Build history of the part. All positions in model axes, mm. Face numbers are marked on the shaded views. A direction names the side the tool comes from. Round coordinates to 2 decimals unless told otherwise and drop trailing zeros. Loops run counter-clockwise (first coordinate to the right, second up) from the corner with the lowest first, then second, coordinate; pieces in that order, holes last. Notation, with made-up numbers: (79, -30) - (102, -30) arc R32 ccw to (102, -3) - close; hole circle Ø8 at (57.25, -31). An arc over 180 degrees is marked (long way). Use one line per item in the form item = value. Start each with the question number.
Q1. Saw through at A-A (x = 0). Give the cut face in (y, z).
Q2. Saw through at D-D (x = 12). Give the cut face in (y, z), then the cut area to 3 significant figures.
Q3. Mould opens along X. For the marked faces 1, 2 and 3 say: released by +X, released by -X, zero draft, split by the parting line, or undercut.
Q4. Saw through at B-B (z = 4). Give the cut face in (x, y).
Q5. Saw through at C-C (y = -9). Give the cut face in (x, z).
Q6. Pin check, flat tips, straight feed: pin 1 (6 mm diameter, centred on x = 32, y = 4.5, fed in from +Z); pin 2 (1 mm diameter, centred on y = -10.5, z = 8.5, fed in from -X); pin 3 (1.5 mm diameter, centred on x = 18, z = 13, fed in from -Y). Stop position of each tip, or through.
Q7. Drill centre lines: line 1 (Z direction, x = -38.5, y = 21.5); line 2 (X direction, y = 3, z = 10.75); line 3 (X direction, y = 16.5, z = 18.5). Where is each one in solid material? Low to high.
Q8. 3-axis set-ups, long thin cutter, end or side, ignore diameter. For the marked faces 4, 5 and 6: which of +Z, -Z, +X, -X, +Y, -Y reach the whole face in a straight line?
```python
from build123d import *

# Parameters (mm, degrees)
SKETCH1_R           = 50.8
BOSS_EXTRUDE1_DEPTH = 6.35
SKETCH2_R           = 19.05
BOSS_EXTRUDE2_DEPTH = 19.05
CUT_EXTRUDE1_DEPTH  = 25.4
SKETCH4_R           = 3.81


with BuildPart() as part:
    # Sketch1 → Boss-Extrude1 (new body)
    with BuildSketch(Plane.XY):
        Circle(SKETCH1_R)
    extrude(amount=BOSS_EXTRUDE1_DEPTH)

    # Sketch2 → Boss-Extrude2 (add)
    with BuildSketch(Plane.XY.offset(6.35)):
        with Locations(Location((0, 0, 0), (0, 0, 180))):
            Circle(SKETCH2_R)
    extrude(amount=BOSS_EXTRUDE2_DEPTH)

    # Sketch3 → Cut-Extrude1 (cut)
    with BuildSketch(Plane.XY.offset(25.4)):
        Polygon((7.332348419, 0), (3.666174209, 6.35), (-3.666174209, 6.35), (-7.332348419, 0), (-3.666174209, -6.35), (3.666174209, -6.35), align=None)
    extrude(amount=-CUT_EXTRUDE1_DEPTH, mode=Mode.SUBTRACT)

    # Sketch4 → Cut-Revolve1 (revolve, cut)
    with BuildSketch(Plane(origin=(0, 19.05, 0), x_dir=(1, 0, 0), z_dir=(0, 1, 0)), mode=Mode.PRIVATE) as cut_revolve1_sk:
        with Locations((0, -19.05)):
            Circle(SKETCH4_R)
    revolve(cut_revolve1_sk.sketch.rotate(Axis((25.4, 19.05, 25.4), (-1, 0, 0)), 45.450641154), axis=Axis((25.4, 19.05, 25.4), (-1, 0, 0)), mode=Mode.SUBTRACT)


solid = part.part
```
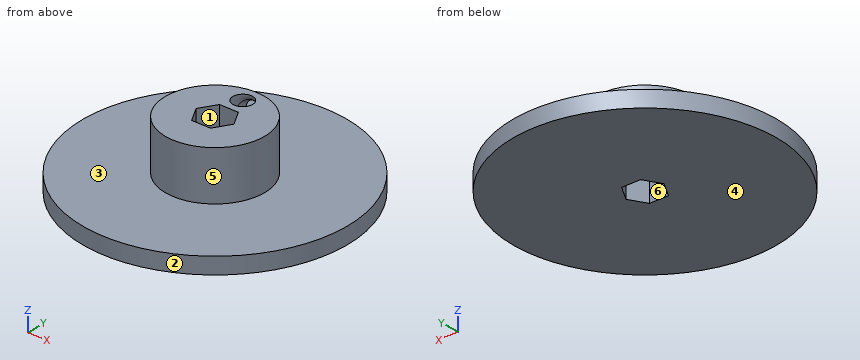
Report:
q1.outline = (-50.8, 0) - (-6.35, 0) - (-6.35, 25.4) - (-19.05, 25.4) - (-19.05, 6.35) - (-50.8, 6.35) - close; (6.35, 0) - (50.8, 0) - (50.8, 6.35) - (19.05, 6.35) - (19.05, 15.24) arc R10.16 cw to (8.89, 25.4) - (6.35, 25.4) - close; (16.51, 25.4) arc R2.54 ccw to (19.05, 22.86) - (19.05, 25.4) - close
q2.outline = (-49.36, 0) - (49.36, 0) - (49.36, 6.35) - (14.8, 6.35) - (14.8, 25.4) - (-14.8, 25.4) - (-14.8, 6.35) - (-49.36, 6.35) - close
q2.area = 1,190 mm²
q3.face_1 = undercut
q3.face_2 = split by the parting line
q3.face_3 = zero draft
q4.outline = circle Ø101.6 at (0, 0); hole (-7.33, 0) - (-3.67, -6.35) - (3.67, -6.35) - (7.33, 0) - (3.67, 6.35) - (-3.67, 6.35) - close
q5.outline = (-50, 0) - (50, 0) - (50, 6.35) - (16.79, 6.35) - (16.79, 25.4) - (-16.79, 25.4) - (-16.79, 6.35) - (-50, 6.35) - close
q6.pin_1 = 6.35
q6.pin_2 = -16.21
q6.pin_3 = -8.08
q7.line_1 = 0 to 6.35
q7.line_2 = -18.81 to -5.6, 5.6 to 18.81
q7.line_3 = -9.52 to -3.67, 3.67 to 9.52
q8.face_4 = -Z, +X, -X, +Y, -Y
q8.face_5 = +Z
q8.face_6 = +Z, -Z
